```python
from build123d import *

# Parameters (mm, degrees)
SKETCH1_W           = 465
SKETCH1_H           = 90
SKETCH1_R           = 2.55
BOSS_EXTRUDE1_DEPTH = 2.2479
CUT_EXTRUDE1_REACH  = 238.857
SKETCH2_R           = 1.6
SKETCH2_W           = 38
SKETCH2_H           = 14


with BuildPart() as part:
    # Sketch1 → Boss-Extrude1 (new, symmetric)
    with BuildSketch(Plane.XY):
        Rectangle(SKETCH1_W, SKETCH1_H)
        with Locations((-222.5, 35)):
            Circle(SKETCH1_R, mode=Mode.SUBTRACT)
        with Locations((-222.5, -35)):
            Circle(SKETCH1_R, mode=Mode.SUBTRACT)
        with Locations((0, 35)):
            Circle(SKETCH1_R, mode=Mode.SUBTRACT)
        with Locations((-114.975, 35)):
            Circle(SKETCH1_R, mode=Mode.SUBTRACT)
        with Locations(Location((222.5, -35, 0), (0, 0, 180))):
            Circle(SKETCH1_R, mode=Mode.SUBTRACT)
        with Locations(Location((222.5, 35, 0), (0, 0, 180))):
            Circle(SKETCH1_R, mode=Mode.SUBTRACT)
        with Locations(Location((114.975, 35, 0), (0, 0, 180))):
            Circle(SKETCH1_R, mode=Mode.SUBTRACT)
    extrude(amount=BOSS_EXTRUDE1_DEPTH, both=True)

    # Sketch2 → Cut-Extrude1 (cut, up to next)
    with BuildSketch(Plane.XY.offset(2.2479), mode=Mode.PRIVATE) as cut_extrude1_sk1:
        with Locations((-6.5, 21)):
            Circle(SKETCH2_R)
    cut_extrude1_tool1 = extrude(cut_extrude1_sk1.sketch, amount=-CUT_EXTRUDE1_REACH, mode=Mode.PRIVATE) & part.part
    # Sketch2 → Cut-Extrude1 (cut, up to next)
    with BuildSketch(Plane.XY.offset(2.2479), mode=Mode.PRIVATE) as cut_extrude1_sk2:
        with Locations((-38.5, 21)):
            Circle(SKETCH2_R)
    cut_extrude1_tool2 = extrude(cut_extrude1_sk2.sketch, amount=-CUT_EXTRUDE1_REACH, mode=Mode.PRIVATE) & part.part
    # Sketch2 → Cut-Extrude1 (cut, up to next)
    with BuildSketch(Plane.XY.offset(2.2479), mode=Mode.PRIVATE) as cut_extrude1_sk3:
        with Locations((-38.5, -11)):
            Circle(SKETCH2_R)
    cut_extrude1_tool3 = extrude(cut_extrude1_sk3.sketch, amount=-CUT_EXTRUDE1_REACH, mode=Mode.PRIVATE) & part.part
    # Sketch2 → Cut-Extrude1 (cut, up to next)
    with BuildSketch(Plane.XY.offset(2.2479), mode=Mode.PRIVATE) as cut_extrude1_sk4:
        with Locations((-6.5, -11)):
            Circle(SKETCH2_R)
    cut_extrude1_tool4 = extrude(cut_extrude1_sk4.sketch, amount=-CUT_EXTRUDE1_REACH, mode=Mode.PRIVATE) & part.part
    # Sketch2 → Cut-Extrude1 (cut, up to next)
    with BuildSketch(Plane.XY.offset(2.2479), mode=Mode.PRIVATE) as cut_extrude1_sk5:
        with Locations((-103.5, 10)):
            Rectangle(SKETCH2_W, SKETCH2_H)
    cut_extrude1_tool5 = extrude(cut_extrude1_sk5.sketch, amount=-CUT_EXTRUDE1_REACH, mode=Mode.PRIVATE) & part.part
    # Sketch2 → Cut-Extrude1 (cut, up to next)
    with BuildSketch(Plane.XY.offset(2.2479), mode=Mode.PRIVATE) as cut_extrude1_sk6:
        Polygon((210.636873287, -8), (199.923313965, 22.1), (171.076686035, 22.1), (160.363126713, -8), (171.076686035, -38.1), (199.923313965, -38.1), align=None)
    cut_extrude1_tool6 = extrude(cut_extrude1_sk6.sketch, amount=-CUT_EXTRUDE1_REACH, mode=Mode.PRIVATE) & part.part
    # Sketch2 → Cut-Extrude1 (cut, up to next)
    with BuildSketch(Plane.XY.offset(2.2479), mode=Mode.PRIVATE) as cut_extrude1_sk7:
        with BuildLine():
            ThreePointArc((-33.527951396, -10.472048604), (-22.5, -14), (-11.472048604, -10.472048604))
            ThreePointArc((-11.472048604, -10.472048604), (-10.035533906, -7.464466094), (-7.027951396, -6.027951396))
            ThreePointArc((-7.027951396, -6.027951396), (-3.5, 5), (-7.027951396, 16.027951396))
            ThreePointArc((-7.027951396, 16.027951396), (-10.035533906, 17.464466094), (-11.472048604, 20.472048604))
            ThreePointArc((-11.472048604, 20.472048604), (-22.5, 24), (-33.527951396, 20.472048604))
            ThreePointArc((-33.527951396, 20.472048604), (-34.964466094, 17.464466094), (-37.972048604, 16.027951396))
            ThreePointArc((-37.972048604, 16.027951396), (-41.5, 5), (-37.972048604, -6.027951396))
            ThreePointArc((-37.972048604, -6.027951396), (-34.964466094, -7.464466094), (-33.527951396, -10.472048604))
        make_face()
    cut_extrude1_tool7 = extrude(cut_extrude1_sk7.sketch, amount=-CUT_EXTRUDE1_REACH, mode=Mode.PRIVATE) & part.part
    add(cut_extrude1_tool1.solids().sort_by_distance((-6.5, 21, 2.2479))[0], mode=Mode.SUBTRACT)
    add(cut_extrude1_tool2.solids().sort_by_distance((-38.5, 21, 2.2479))[0], mode=Mode.SUBTRACT)
    add(cut_extrude1_tool3.solids().sort_by_distance((-38.5, -11, 2.2479))[0], mode=Mode.SUBTRACT)
    add(cut_extrude1_tool4.solids().sort_by_distance((-6.5, -11, 2.2479))[0], mode=Mode.SUBTRACT)
    add(cut_extrude1_tool5.solids().sort_by_distance((-103.5, 10, 2.2479))[0], mode=Mode.SUBTRACT)
    add(cut_extrude1_tool6.solids().sort_by_distance((185.5, -8, 2.2479))[0], mode=Mode.SUBTRACT)
    add(cut_extrude1_tool7.solids().sort_by_distance((-22.5, 5, 2.2479))[0], mode=Mode.SUBTRACT)


solid = part.part
```
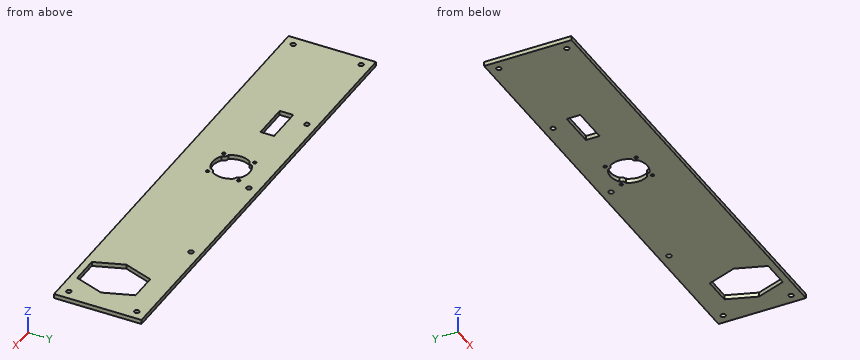
The listing builds one solid part. Answer for the finished solid, in the listing's coordinates (mm). Give positions to 0.01 mm unless a question says otherwise; leave off trailing zeros. Order: outer loops, then holes, each group sorted by start corner. A loop starts at its lowest first (then second) coordinate and runs counter-clockwise, first axis right, second up. Notation, with made-up numbers: (-22.5, 46) -> (1.5, 46) arc R25 cw to (1.5, 62) -> close; hole circle Ø10 at (74.5, -15.75). An arc over 180 degrees is marked (long way). One line per item, written item: value.
1) Find section A-A, the plane x = 184. Determine the outline of the cut face in (y, z).
Reported:
outline: (-45, -2.25) -> (-38.1, -2.25) -> (-38.1, 2.25) -> (-45, 2.25) -> close; (22.1, -2.25) -> (45, -2.25) -> (45, 2.25) -> (22.1, 2.25) -> close
2) Find the intervals of material crossed by line 1 (Y direction, x = 222.5, z = -1.05); line 2 (Y direction, x = -6.5, z = -1.3); line 3 (X direction, y = 33.5, z = 0.2), in increasing order.
Reported:
line 1: y = -45 to -37.55, -32.45 to 32.45, 37.55 to 45
line 2: y = -45 to -12.6, -9.4 to -5.25, 15.25 to 19.4, 22.6 to 45
line 3: x = -232.5 to -224.56, -220.44 to -117.04, -112.91 to -2.06, 2.06 to 112.91, 117.04 to 220.44, 224.56 to 232.5
3) Flat-ended cylindrical pins translate along their axes: P1, Ø5, axis at x = -38.5, y = 21, coming from the -Z side; P2, Ø4, axis at x = -222.5, y = -35, coming from the -Z side. Find the tip coordinate at first contact, or state that the pin passes through.
Reported:
P1: stops at z = -2.25
P2: passes through
4) Find section B-B, the plane z = -1.1. Count the separate pieces of the cut face and the enclosed holes in it, plus the area to 3 significant figures.
Reported:
separate pieces: 1
enclosed holes: 14
area: 37,700 mm^2
5) Find section C-C, the plane y = 8. Determine the outline of the cut face in (x, z), plus the area to 3 significant figures.
Reported:
outline: (-232.5, -2.25) -> (-122.5, -2.25) -> (-122.5, 2.25) -> (-232.5, 2.25) -> close; (-84.5, -2.25) -> (-41.26, -2.25) -> (-41.26, 2.25) -> (-84.5, 2.25) -> close; (-3.74, -2.25) -> (166.06, -2.25) -> (166.06, 2.25) -> (-3.74, 2.25) -> close; (204.94, -2.25) -> (232.5, -2.25) -> (232.5, 2.25) -> (204.94, 2.25) -> close
area: 1,580 mm^2
